For this review, take the finished solid that the model builds, in its own axes (mm). Face numbers are marked on the shaded views. A direction names the side the tool comes from. Give positions to 0.01 mm unless a question says otherwise; leave off trailing zeros. Order: outer loops, then holes, each group sorted by start corner. A loop starts at its lowest first (then second) coordinate and runs counter-clockwise, first axis right, second up. Notation, with made-up numbers: (50.25, -8.5) - (85.25, -8.5) arc R25 ccw to (85.25, 18.5) - close; hole circle Ø2 at (5.5, 46.25). An arc over 180 degrees is marked (long way). Answer as a JSON object with one key per item and string values. Group by question number.
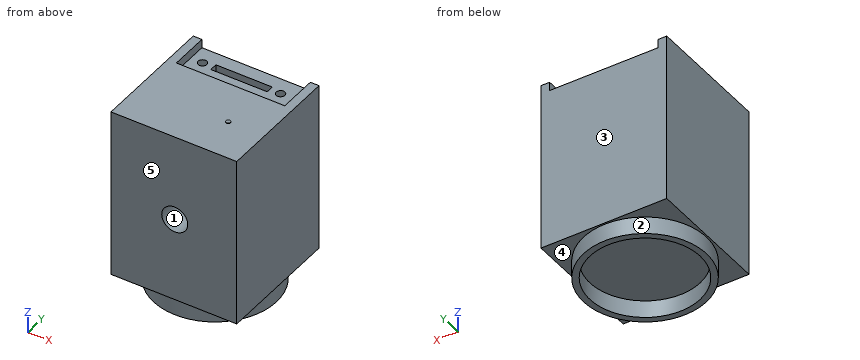
from build123d import *

# Parameters (mm, degrees)
SKETCH2_W           = 29
SKETCH2_H           = 29
BOSS_EXTRUDE1_DEPTH = 39.3
SKETCH3_R           = 14.15
SKETCH3_R_2         = 12.7
BOSS_EXTRUDE2_DEPTH = 4
SKETCH4_W           = 25
SKETCH4_H           = 9
CUT_EXTRUDE1_DEPTH  = 2
SKETCH5_R           = 1
SKETCH5_W           = 13
SKETCH5_H           = 1.8
CUT_EXTRUDE2_DEPTH  = 5
SKETCH6_R           = 0.517544676
BOSS_EXTRUDE3_DEPTH = 0.1
SKETCH7_R           = 3
CUT_EXTRUDE3_DEPTH  = 7


with BuildPart() as part:
    # Sketch2 → Boss-Extrude1 (new body)
    with BuildSketch(Plane.XY):
        with Locations((-23.624610592, 3.658878505)):
            Rectangle(SKETCH2_W, SKETCH2_H)
    extrude(amount=BOSS_EXTRUDE1_DEPTH)

    # Sketch3 → Boss-Extrude2 (add)
    with BuildSketch(Plane(origin=(0, 0, 0), x_dir=(-1, 0, 0), z_dir=(0, 0, -1))):
        with Locations(Location((23.624610592, 3.658878505, 0), (0, 0, 180))):
            Circle(SKETCH3_R)
        with Locations((23.624610592, 3.658878505)):
            Circle(SKETCH3_R_2, mode=Mode.SUBTRACT)
    extrude(amount=BOSS_EXTRUDE2_DEPTH)

    # Sketch4 → Cut-Extrude1 (cut)
    with BuildSketch(Plane.XY.offset(39.3)):
        with Locations((-23.624610592, 13.658878505)):
            Rectangle(SKETCH4_W, SKETCH4_H)
    extrude(amount=-CUT_EXTRUDE1_DEPTH, mode=Mode.SUBTRACT)

    # Sketch5 → Cut-Extrude2 (cut)
    with BuildSketch(Plane.XY.offset(37.3)):
        with Locations((-33.374610592, 14.158878505)):
            Circle(SKETCH5_R)
        with Locations((-15.374610592, 14.158878505)):
            Circle(SKETCH5_R)
        with Locations((-24.374610592, 14.158878505)):
            Rectangle(SKETCH5_W, SKETCH5_H)
    extrude(amount=-CUT_EXTRUDE2_DEPTH, mode=Mode.SUBTRACT)

    # Sketch6 → Boss-Extrude3 (add)
    with BuildSketch(Plane.XY.offset(39.3)):
        with Locations((-17.424610592, -1.141121495)):
            Circle(SKETCH6_R)
    extrude(amount=BOSS_EXTRUDE3_DEPTH)

    # Sketch7 → Cut-Extrude3 (cut)
    with BuildSketch(Plane.XZ.offset(10.841121495)):
        with Locations(Location((-23.417250102, 19.368990784, 0), (0, 0, 270))):
            Circle(SKETCH7_R)
    extrude(amount=-CUT_EXTRUDE3_DEPTH, mode=Mode.SUBTRACT)


solid = part.part
1) Mouldability with a two-part tool opening along X and no side actions: class the marked faces 1, 2 and 3 as released by +X, released by -X, zero draft, split by the parting line, or undercut.
2) Consider section A-A (y = -6.25). Give the boundary of the cut face in (x, z).
3) For pin 1 (10 mm diameter, centred on x = -25, y = 15, fed in from +Z); pin 2 (1 mm diameter, centred on x = -29.5, z = 38, fed in from +Y); pin 3 (3 mm diameter, centred on x = -24.5, y = -6.5, fed in from -Z), all flat-tipped, find the tip position at first contact; note any pin that passes through.
4) Consider section D-D (y = 0). Give the boundary of the cut face in (x, z), plus the area to 3 significant figures.
5) For the marked faces 4 and 5, list the 3-axis set-ups (+Z, -Z, +X, -X, +Y, -Y) from which the entire face can be reached by the end or side of a thin tool; tool diameter is ignored.
6) For line 1 (Z direction, x = -37, y = 15); line 2 (Z direction, x = -25.25, y = -4.5); line 3 (Z direction, x = -22.25, y = 11.5), list the stretches that pass through material, from the lowest coordinate up.
7) Consider section B-B (x = -28.5). Give the boundary of the cut face in (y, z).
8) Consider section C-C (z = 17.5). Give the boundary of the cut face in (x, y), plus the area to 3 significant figures.
Result set:
{
 "1": {"face 1": "undercut", "face 2": "split by the parting line", "face 3": "zero draft"},
 "2": {"outline": "(-38.12, 0) - (-33.73, 0) - (-33.73, -4) - (-31.57, -4) - (-31.57, 0) - (-15.68, 0) - (-15.68, -4) - (-13.52, -4) - (-13.52, 0) - (-9.12, 0) - (-9.12, 39.3) - (-38.12, 39.3) - close; hole circle Ø6 at (-23.42, 19.37)"},
 "3": {"pin 1": "stops at z = 37.3", "pin 2": "stops at y = 9.16", "pin 3": "stops at z = 0"},
 "4": {"outline": "(-38.12, 0) - (-37.29, 0) - (-37.29, -4) - (-35.79, -4) - (-35.79, 0) - (-11.46, 0) - (-11.46, -4) - (-9.96, -4) - (-9.96, 0) - (-9.12, 0) - (-9.12, 39.3) - (-38.12, 39.3) - close", "area": "1,150 mm2"},
 "5": {"face 4": "-Z", "face 5": "+Z, -Z, +X, -X, -Y"},
 "6": {"line 1": "z = 0 to 39.3", "line 2": "z = 0 to 16.99, 21.74 to 39.3", "line 3": "z = 0 to 37.3"},
 "7": {"outline": "(-10.84, 0) - (-9.62, 0) - (-9.62, -4) - (-8.07, -4) - (-8.07, 0) - (15.39, 0) - (15.39, -4) - (16.94, -4) - (16.94, 0) - (18.16, 0) - (18.16, 37.3) - (15.06, 37.3) - (15.06, 32.3) - (13.26, 32.3) - (13.26, 37.3) - (9.16, 37.3) - (9.16, 39.3) - (-10.84, 39.3) - close"},
 "8": {"outline": "(-38.12, -10.84) - (-25.76, -10.84) - (-25.76, -3.84) - (-21.07, -3.84) - (-21.07, -10.84) - (-9.12, -10.84) - (-9.12, 18.16) - (-38.12, 18.16) - close", "area": "808 mm2"}
}
